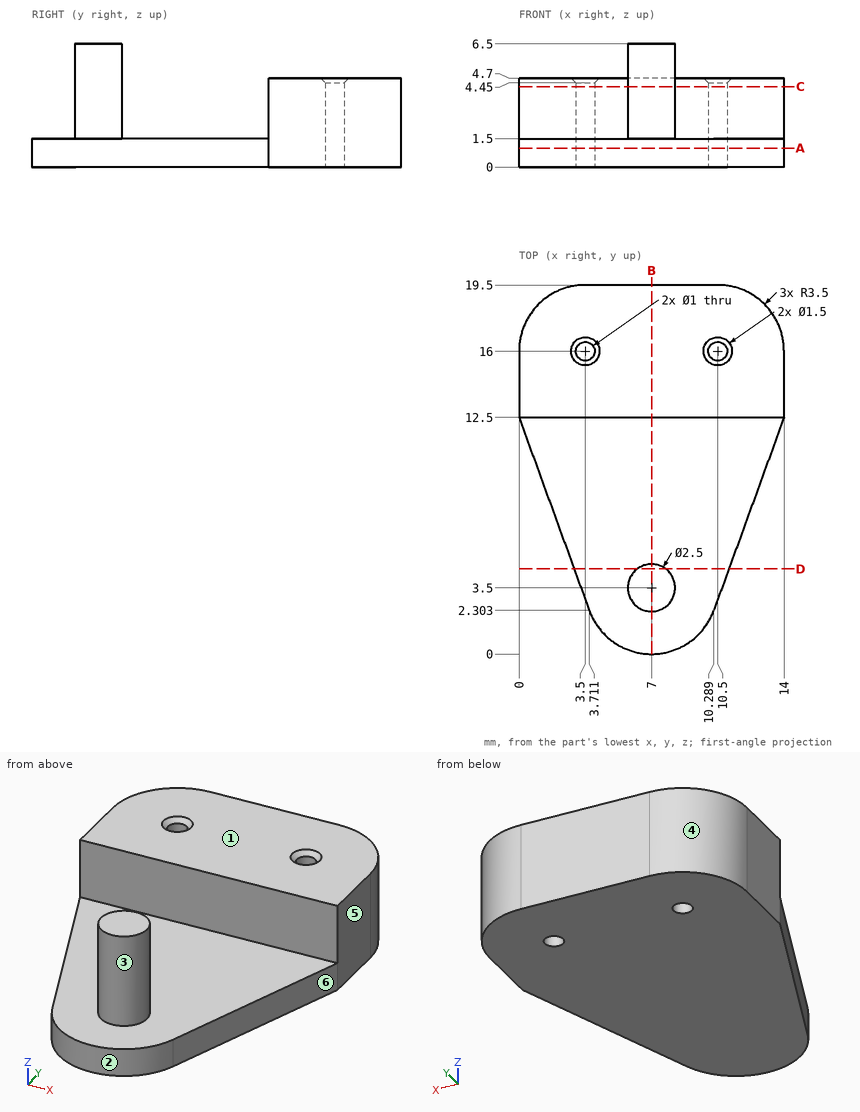
Geometry check sheet. Reference: drawing and pictorial views, mm from the part's lowest x, y, z. A direction names the side the tool comes from. Coordinates: 2 decimals unless noted, no trailing zeros. Write each loop counter-clockwise with the first axis right and the second up, starting at its lowest first coordinate (ties: lowest second). Pieces come first, ordered by that corner, then holes.
Item 1: Cross-section at A-A on z = 1. Record the boundary of the cut face in (x, y), then the cut area to 3 significant figures.
Numbers:
outline: (0, 12.5) - (3.71, 2.3) arc R3.5 ccw to (10.29, 2.3) - (14, 12.5) - (14, 16) arc R3.5 ccw to (10.5, 19.5) - (3.5, 19.5) arc R3.5 ccw to (0, 16) - close; hole circle Ø1 at (3.5, 16); hole circle Ø1 at (10.5, 16)
area: 207 mm2
Item 2: Scan lines: probe 1 along Y at (x, z) = (10.5, 2.1); probe 2 along Z at (x, y) = (10, 6); probe 3 along Z at (x, y) = (12.75, 17.5). Record each from-to range of solid material in increasing order.
Numbers:
probe 1: y = 12.5 to 15.5, 16.5 to 19.5
probe 2: z = 0 to 1.5
probe 3: z = 0 to 4.7
Item 3: Cross-section at B-B on x = 7. Record the boundary of the cut face in (y, z).
Numbers:
outline: (0, 0) - (19.5, 0) - (19.5, 4.7) - (12.5, 4.7) - (12.5, 1.5) - (4.75, 1.5) - (4.75, 6.5) - (2.25, 6.5) - (2.25, 1.5) - (0, 1.5) - close
Item 4: Cross-section at D-D on y = 4.5. Record the boundary of the cut face in (x, z).
Numbers:
outline: (2.91, 0) - (11.09, 0) - (11.09, 1.5) - (7.75, 1.5) - (7.75, 6.5) - (6.25, 6.5) - (6.25, 1.5) - (2.91, 1.5) - close
Item 5: Depth check by flat-ended pin: pin 1 Ø1 at (x, z) = (8.5, 3) entering from -Y; pin 2 Ø1 at (x, y) = (6, 15.5) entering from +Z. Enter the tip coordinate at first touch or a pass-through.
Numbers:
pin 1: stops at y = 2.75
pin 2: stops at z = 4.7
Item 6: Cross-section at C-C on z = 4.25. Record the boundary of the cut face in (x, y).
Numbers:
outline: (0, 12.5) - (14, 12.5) - (14, 16) arc R3.5 ccw to (10.5, 19.5) - (3.5, 19.5) arc R3.5 ccw to (0, 16) - close; circle Ø2.5 at (7, 3.5); hole circle Ø1 at (3.5, 16); hole circle Ø1 at (10.5, 16)
Item 7: Access from +Z, -Z, +X, -X, +Y, -Y to the whole of each face (thin tool, end or side, straight path). Record for the marked faces 1 and 2.
Numbers:
face 1: +Z, +X, -X, +Y
face 2: +Z, -Z, -Y
Item 8: Mould release check, pull along Y, two halves, no side actions. Record for the marked faces 3, 4, 5 and 6: released by +Y, released by -Y, zero draft, split by the parting line, or undercut.
Numbers:
face 3: undercut
face 4: released by +Y
face 5: zero draft
face 6: released by -Y
